Autodesk Inventor part; units mm, degrees
ref_plane "YZ Plane" through (0, 0, 0) normal (1, 0, 0) x (0, 1, 0)
ref_plane "XZ Plane" through (0, 0, 0) normal (0, 1, 0) x (-1, 0, 0)
ref_plane "XY Plane" through (0, 0, 0) normal (0, 0, 1) x (1, 0, 0)
sketch "Sketch1" plane through (0, 0, 0) normal (0, 1, 0) x (-1, 0, 0)
  circle A0 centre (0, 0) radius 5
  dimension "d0" = 10
extrude "Extrusion1" add sketch "Sketch1" along normal blind 80
sketch "Sketch2" plane through (0, 0, 0) normal (0, 0, 1) x (1, 0, 0)
  circle A0 centre (0, 20) radius 1
  point P0 (0, 0)
  dimension "d3" = 2
extrude "Extrusion2" add sketch "Sketch2" against normal mid plane 10
sketch "Sketch3" plane through (0, 80, 0) normal (0, 1, 0) x (1, 0, 0)
  circle A0 centre (0, 0) radius 2.5
  dimension "d6" = 5
extrude "Extrusion3" cut sketch "Sketch3" against normal through all keep common part
Part model, mm, in its own coordinate system. Round coordinates to 2 decimals unless told otherwise and drop trailing zeros. Loops run counter-clockwise (first coordinate to the right, second up) from the corner with the lowest first, then second, coordinate; pieces in that order, holes last. Notation, with made-up numbers: (13, 41) - (34, 41) arc R24 ccw to (34, 51) - close; hole circle Ø1 at (18, 81). An arc over 180 degrees is marked (long way). Answer as a JSON object with one key per item and string values.
Item 1: Band-saw the part on A-A on z = 0.7. List the corners of the cut face in (x, y), plus the area to 3 significant figures.
Output:
{"outline": "(-2.4, 0) - (2.4, 0) - (2.4, 80) - (-2.4, 80) - close", "area": "384 mm2"}
Item 2: Band-saw the part on B-B on y = 18. List the corners of the cut face in (x, z), plus the area to 3 significant figures.
Output:
{"outline": "circle Ø5 at (0, 0)", "area": "19.6 mm2"}
Item 3: Wall check: L1, parallel to Z at x = -0.1, y = 32; L2, parallel to X at y = 59.5, z = -1.25. Give the ranges that are in metal, low to high.
Output:
{"L1": "-2.5 to 2.5", "L2": "-2.17 to 2.17"}
Item 4: Band-saw the part on C-C on x = 1.2. List the corners of the cut face in (y, z).
Output:
{"outline": "(0, -2.19) - (80, -2.19) - (80, 2.19) - (0, 2.19) - close"}
